For this review, take the finished solid that the model builds, in its own axes (mm). A direction names the side the tool comes from. Round coordinates to 2 decimals unless told otherwise and drop trailing zeros. Write each loop counter-clockwise with the first axis right and the second up, starting at its lowest first coordinate (ties: lowest second). Pieces come first, ordered by that corner, then holes. Notation, with made-up numbers: (-4, -12.75) - (40, -12.75) arc R11 ccw to (40, -4.75) - close; hole circle Ø3 at (-27.75, 48.5). An arc over 180 degrees is marked (long way). One line per item, written item: value. Start each with the question number.
Q1. For probe 1 along Z at (x, y) = (0, -10.5); probe 2 along Y at (x, z) = (2.75, 0.5); probe 3 along Z at (x, y) = (-0.25, -2.5), list the stretches that pass through material, from the lowest coordinate up.
Q2. Tool access review of faces 5 (the face through (-0.76, -0.986, 1.293)), 6 (the face through (-2, 0, 0)): name each direction out of +Z, -Z, +X, -X, +Y, -Y from which nothing blocks a thin tool from reaching the whole face with its end or side.
Q3. Clearance check with flat-ended pins moving along their axes: pin 1 Ø0.6 at (x, z) = (1, -0.5) entering from +Y; pin 2 Ø2 at (y, z) = (-6.5, 2) entering from +X; pin 3 Ø1.5 at (y, z) = (-11.5, 0) entering from +X; pin 4 Ø3 at (x, z) = (-1, -2) entering from +Y. State where each tip first meets the part, or that it passes through.
Q4. Add section B-B on x = -2.5. Write out the cut boundary in (y, z).
Q5. Mouldability with a two-part tool opening along Z and no side actions: class faces 1 (the face through (0, -9, -2)), 2 (the face through (0.76, -0.986, -1.293)), 3 (the face through (1.5, -1, 0)), 4 (the face through (2, -4, -2)) as +Z half, -Z half, draft (parallel to the pull), parting line (faces both ways), or undercut.
Q6. Add section A-A on y = -9. Write out the cut boundary in (x, z), and give its area (3 significant figures).
```python
from build123d import *

# Parameters (mm, degrees)
CUT_EXTRUDE1_DEPTH = 2


with BuildPart() as part:
    # Sketch1 → Revolve1 (revolve)
    with BuildSketch(Plane.XY):
        Polygon((0, 0), (3.5, 0), (3.5, -4), (2, -4), (2, -14), (0, -14), align=None)
    revolve(axis=Axis((0, 0, 0), (0, -1, 0)))

    # Sketch2 → Cut-Revolve1 (revolve, cut)
    with BuildSketch(Plane.XY):
        Polygon((1.5, 0), (1.5, -2), (0, -2.866025404), (0, 0), align=None)
    revolve(axis=Axis((0, 0, 0), (0, -1, 0)), mode=Mode.SUBTRACT)

    # Sketch3 → Cut-Extrude1 (cut)
    with BuildSketch(Plane(origin=(0, 0, 0), x_dir=(1, 0, 0), z_dir=(0, 1, 0))):
        Polygon((0, 1.732050808), (-1.5, 0.866025404), (-1.5, -0.866025404), (0, -1.732050808), (1.5, -0.866025404), (1.5, 0.866025404), align=None)
    extrude(amount=-CUT_EXTRUDE1_DEPTH, mode=Mode.SUBTRACT)


solid = part.part
```
Result set:
1. probe 1: z = -2 to 2
1. probe 2: y = -4 to 0
1. probe 3: z = -3.49 to -0.58, 0.58 to 3.49
2. face 5: +Y
2. face 6: +Z, -Z, +X, -X, +Y
3. pin 1: stops at y = -2.05
3. pin 2: stops at x = 1.73
3. pin 3: stops at x = 2
3. pin 4: stops at y = 0
4. outline: (-4, -2.45) - (0, -2.45) - (0, 2.45) - (-4, 2.45) - close
5. face 1: parting line
5. face 2: undercut
5. face 3: undercut
5. face 4: draft
6. outline: circle Ø4 at (0, 0)
6. area: 12.6 mm^2
